For this review, take the finished solid that the model builds, in its own axes (mm). A direction names the side the tool comes from. Coordinates: 2 decimals unless noted, no trailing zeros. Loops run counter-clockwise (first coordinate to the right, second up) from the corner with the lowest first, then second, coordinate; pieces in that order, holes last. Notation, with made-up numbers: (69, 6) - (98, 6) arc R31 ccw to (98, 44) - close; hole circle Ø11 at (-27.5, 82). An arc over 180 degrees is marked (long way). One line per item, written item: value. Start each with the question number.
1. The part is to be moulded in two halves that separate along X. For faces 1 (the face through (-1, 0, 3)), 2 (the face through (-33, 3.25, 1)), 3 (the face through (23, -23.25, 1)), say which applies: released by +X, released by -X, zero draft, split by the parting line, or undercut.
2. Take a section at C-C, the plane x = 6.5. State the section outline as (y, z) points, and give its area (3 significant figures).
3. To check wall thickness, follow line 1 (Y direction, x = -11, z = 1.4); line 2 (X direction, y = -26, z = 0.9); line 3 (X direction, y = 13.5, z = 2.3). State the ranges of each line that lie inside material, in increasing order. Write a range as from..to.
4. Insertion check: pin 1 (2.5 mm diameter, centred on x = -23.5, y = 0, fed in from -Z). The pin has a flat end and moves straight along its axis. Give the tip position at first contact, or say it passes through.
5. For faces 4 (the face through (-1, -30, 1)), 5 (the face through (-8, -3.25, 1)), list the 3-axis set-ups (+Z, -Z, +X, -X, +Y, -Y) from which the entire face can be reached by the end or side of a thin tool; tool diameter is ignored.
6. Take a section at B-B, the plane y = 26. State the section outline as (x, z) points.
7. Take a section at A-A, the plane x = -7.5. State the section outline as (y, z) points, and give its area (3 significant figures).
8. Take a section at D-D, the plane z = 2.25. Count the separate pieces of the cut face and the enclosed holes in it, and give its area (3 significant figures).
```python
from build123d import *

# Parameters (mm, degrees)
SKETCH1_W           = 100
SKETCH1_H           = 60
BOSS_EXTRUDE1_DEPTH = 3
SKETCH3_R           = 1.5
SKETCH3_R_2         = 2
CUT_EXTRUDE2_DEPTH  = 10


with BuildPart() as part:
    # Sketch1 → Boss-Extrude1 (new body)
    with BuildSketch(Plane.XY):
        Rectangle(SKETCH1_W, SKETCH1_H)
    extrude(amount=BOSS_EXTRUDE1_DEPTH)

    # Sketch3 → Cut-Extrude2 (cut)
    with BuildSketch(Plane(origin=(0, 0, 0), x_dir=(-1, 0, 0), z_dir=(0, 0, -1))):
        with Locations((43.333333333, 26)):
            Circle(SKETCH3_R)
        with Locations((-43.333333333, 26)):
            Circle(SKETCH3_R)
        with Locations((23.5, 0)):
            Circle(SKETCH3_R_2)
        with Locations((-6.5, 0)):
            Circle(SKETCH3_R_2)
        with Locations((43.5, 0)):
            Circle(SKETCH3_R_2)
        with BuildLine():
            Line((29.129165125, 3.25), (37.870834875, 3.25))
            ThreePointArc((37.870834875, 3.25), (40.25, 5.629165125), (43.5, 6.5))
            Line((43.5, 6.5), (43.5, 18.0017363))
            ThreePointArc((43.5, 18.0017363), (38.819316651, 19.395179534), (35.820843733, 23.25))
            Line((35.820843733, 23.25), (26.75, 23.25))
            Line((26.75, 23.25), (26.75, 5.629165125))
            ThreePointArc((26.75, 5.629165125), (28.096194078, 4.596194078), (29.129165125, 3.25))
        make_face()
        with BuildLine():
            Line((-9.75, 23.25), (-35.820843733, 23.25))
            ThreePointArc((-35.820843733, 23.25), (-38.819316651, 19.395179534), (-43.5, 18.0017363))
            Line((-43.5, 18.0017363), (-43.5, 3.25))
            Line((-43.5, 3.25), (-12.129165125, 3.25))
            ThreePointArc((-12.129165125, 3.25), (-11.096194078, 4.596194078), (-9.75, 5.629165125))
            Line((-9.75, 5.629165125), (-9.75, 23.25))
        make_face()
        with BuildLine():
            Line((-0.870834875, 3.25), (17.870834875, 3.25))
            ThreePointArc((17.870834875, 3.25), (18.903805922, 4.596194078), (20.25, 5.629165125))
            Line((20.25, 5.629165125), (20.25, 23.25))
            Line((20.25, 23.25), (-3.25, 23.25))
            Line((-3.25, 23.25), (-3.25, 5.629165125))
            ThreePointArc((-3.25, 5.629165125), (-1.903805922, 4.596194078), (-0.870834875, 3.25))
        make_face()
    cut_extrude2 = extrude(amount=-CUT_EXTRUDE2_DEPTH, mode=Mode.SUBTRACT)

    # Mirror3: Cut-Extrude2 across plane
    add(cut_extrude2.mirror(Plane.ZX), mode=Mode.SUBTRACT)


solid = part.part
```
Solutions:
1. face 1: zero draft
1. face 2: undercut
1. face 3: undercut
2. outline: (-30, 0) - (-2, 0) - (-2, 3) - (-30, 3) - close; (2, 0) - (30, 0) - (30, 3) - (2, 3) - close
2. area: 168 mm2
3. line 1: -30..-23.25, -3.25..3.25, 23.25..30
3. line 2: -50..-44.83, -41.83..41.83, 44.83..50
3. line 3: -50..-43.5, -26.75..-20.25, 3.25..9.75, 43.5..50
4. pin 1: through
5. face 4: +Z, -Z, +X, -X, -Y
5. face 5: +Z, -Z
6. outline: (-50, 0) - (-44.83, 0) - (-44.83, 3) - (-50, 3) - close; (-41.83, 0) - (41.83, 0) - (41.83, 3) - (-41.83, 3) - close; (44.83, 0) - (50, 0) - (50, 3) - (44.83, 3) - close
7. outline: (-30, 0) - (-23.25, 0) - (-23.25, 3) - (-30, 3) - close; (-3.25, 0) - (3.25, 0) - (3.25, 3) - (-3.25, 3) - close; (23.25, 0) - (30, 0) - (30, 3) - (23.25, 3) - close
7. area: 60.0 mm2
8. separate pieces: 1
8. enclosed holes: 13
8. area: 3,140 mm2
